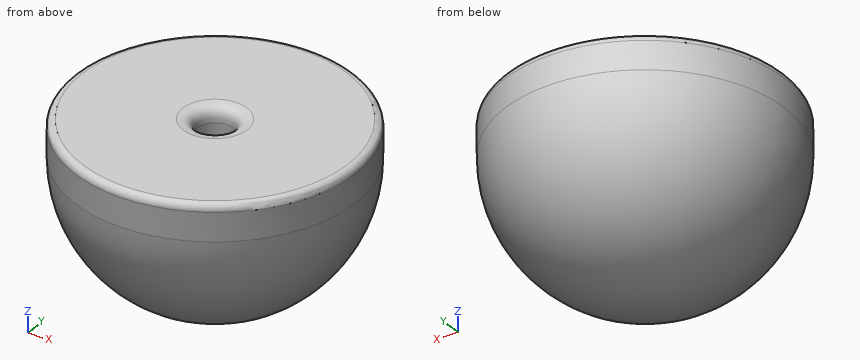
from build123d import *

# Parameters (mm, degrees)
F2_R     = 49.784
F2_R_2   = 6.35
F3_DEPTH = 12.7
F4_R     = 2.54
F6_DEPTH = 15.24
F7_R     = 1.27


# Not quite as in the source:
# - a fillet or chamfer that OpenCascade refuses, or shapes differently, is made with other operations: its cross-section is extruded or revolved along the edge and cut away or added


with BuildPart() as f1:
    # F0 (on Front) → F1 (revolve)
    with BuildSketch(Plane.XZ):
        with BuildLine():
            Line((0, 0), (-49.784, 0))
            ThreePointArc((-49.784, 0), (-35.2026039946, -35.2026039946), (0, -49.784))
            Line((0, -49.784), (0, 0))
        make_face()
    revolve(axis=Axis((0, 0, -24.892), (0, 0, -1)))

    # F2 (on face) → F3 (join)
    with BuildSketch(Plane.XY):
        Circle(F2_R)
        Circle(F2_R_2, mode=Mode.SUBTRACT)
    extrude(amount=F3_DEPTH)

    # F4
    f4_edges = [f1.edges().sort_by_distance(p)[0] for p in [
        (-49.784, 0, 12.7),
    ]]
    fillet(f4_edges, radius=F4_R)

    # F5: fillet of radius 5.08 on 1 edges, made by hand

    # F5_s1 → F5_t2 (revolve, cut)
    with BuildSketch(Plane.XZ):
        with BuildLine():
            add(Edge.make_bspline(
                [(11.43, 12.7), (6.35, 12.7), (6.35, 7.62)],
                knots=[0, 0, 0, 1, 1, 1], degree=2, weights=[1, 1, 1]))
            Line((6.35, 7.62), (6.35, 12.7))
            Line((6.35, 12.7), (11.43, 12.7))
        make_face()
    revolve(axis=Axis((0, 0, 12.7), (0, 0, 1)), mode=Mode.SUBTRACT)

    # F6 (cut): a face of the model
    f6_faces = [f1.faces().sort_by_distance(p)[0] for p in [
        (0, 0, 0),
    ]]
    extrude(f6_faces, amount=-F6_DEPTH, mode=Mode.SUBTRACT)

    # F7
    f7_edges = [f1.edges().sort_by_distance(p)[0] for p in [
        (-6.35, 0, -15.24),
    ]]
    fillet(f7_edges, radius=F7_R)


solid = f1.part
Could you check a few things on this model? Use its own coordinates, in mm. Give positions to 0.01 mm unless a question says otherwise; leave off trailing zeros. Order: outer loops, then holes, each group sorted by start corner. A loop starts at its lowest first (then second) coordinate and runs counter-clockwise, first axis right, second up.
Item 1: I need wall thicknesses on line 1 (Y direction, x = 0, z = 0); line 2 (Y direction, x = 0, z = -6); line 3 (X direction, y = 30, z = -17). Which ranges of each line are inside material? Lowest first, please.
Item 2: I'm going to push flat-ended pins straight in: pin 1 (2 mm diameter, centred on y = -12.5, z = -14.5, fed in from -X); pin 2 (8 mm diameter, centred on y = 29.5, z = -38.5, fed in from -X); pin 3 (2 mm diameter, centred on y = -13.5, z = -38.5, fed in from +X). Where does each tip first touch, or does it pass through?
Item 3: If we section it at B-B, the plane z = -25: Write out the boundary of the cut face in (x, y), plus the area to 3 significant figures.
Item 4: If we section it at C-C, the plane z = -18: Write out the boundary of the cut face in (x, y).
Item 5: If we section it at A-A, the plane z = 4.5: Write out the boundary of the cut face in (x, y).
Values:
1. line 1: y = -49.78 to -6.35, 6.35 to 49.78
1. line 2: y = -49.42 to -6.35, 6.35 to 49.42
1. line 3: x = -35.91 to 35.91
2. pin 1: stops at x = -46.36
2. pin 2: stops at x = -22.32
2. pin 3: stops at x = 29.91
3. outline: circle Ø86.1 at (0, 0)
3. area: 5,820 mm2
4. outline: circle Ø92.83 at (0, 0)
5. outline: circle Ø99.57 at (0, 0); hole circle Ø12.7 at (0, 0)
